Design review of the part built by this model. Coordinates are the model's own, in mm. A direction names the side the tool comes from. Coordinates: 2 decimals unless noted, no trailing zeros. Loops run counter-clockwise (first coordinate to the right, second up) from the corner with the lowest first, then second, coordinate; pieces in that order, holes last. Notation, with made-up numbers: (10, -35.5) - (28, -35.5) arc R21 cw to (28, -20.5) - close; hole circle Ø2 at (41.5, 84). An arc over 180 degrees is marked (long way). Use one line per item in the form item = value. Start each with the question number.
(1) Clearance check with flat-ended pins moving along their axes: pin 1 Ø2 at (y, z) = (1, -17.5) entering from -X; pin 2 Ø2.5 at (x, z) = (20, -113.24) entering from +Y; pin 3 Ø2 at (x, y) = (-18, 2.5) entering from -Z; pin 4 Ø2 at (y, z) = (2.5, -68.5) entering from +X. State where each tip first meets the part, or that it passes through.
(2) Tool access review of faces 1 (the face through (-5.384, 1.972, -121.458)), 2 (the face through (-13.09, 1.97, -1.18)): name each direction out of +Z, -Z, +X, -X, +Y, -Y from which nothing blocks a thin tool from reaching the whole face with its end or side.
(3) Add section B-B (y = 1.1). Count the separate pieces of the cut face and the enclosed holes in it, plus the area to 3 significant figures.
(4) For L1, parallel to X at y = 0.75, z = -66.5; L2, parallel to X at y = 1.95, z = -68.5; L3, parallel to X at y = 0.8, z = -113, list the stretches that pass through material, from the lowest coordinate up.
(5) Add section A-A (z = -79.5). State the section outline as (x, y) points, plus the area to 3 significant figures.
(6) The part is to be moulded in two halves that separate along Z. For faces 3 (the face through (20.922, 1.972, -122.293)), 4 (the face through (8.213, 1.972, -107.86)), 5 (the face through (-23.97, 1.97, -115.82)), 6 (the face through (4.98, 1.97, -43.79)), say which applies: pulls with the +Z half, pulls with the -Z half, needs draft (parallel to the pull), parting line crosses it, or undercut.
```python
from build123d import *

# Parameters (mm, degrees)
BOSS_EXTRUDE1_DEPTH  = 4
M3_CLEARANCE_HOLE1_D = 3.4
SKETCH4_R            = 1.5
CUT_EXTRUDE1_DEPTH   = 135.330995523


with BuildPart() as part:
    # Sketch1 → Boss-Extrude1 (new body)
    with BuildSketch(Plane(origin=(0, 0, 0), x_dir=(1, 0, 0), z_dir=(0, 1, 0))):
        with BuildLine():
            Line((-9.515488572, 0), (9.515488572, 0))
            ThreePointArc((9.515488572, 0), (13.049333225, 1.15108858), (15.227255138, 4.162686012))
            Line((15.227255138, 4.162686012), (21.674585029, 24.205881435))
            ThreePointArc((21.674585029, 24.205881435), (21.904821248, 25.210967753), (21.959569126, 26.240632696))
            Line((21.959569126, 26.240632696), (20.905492982, 58.256025321))
            Line((20.905492982, 58.256025321), (21.026416806, 91.49070067))
            Line((21.026416806, 91.49070067), (23.354507229, 113.886787435))
            ThreePointArc((23.354507229, 113.886787435), (23.340591043, 115.249277617), (23.019622055, 116.573495146))
            Line((23.019622055, 116.573495146), (18.764127525, 128.174177455))
            ThreePointArc((18.764127525, 128.174177455), (16.566422509, 131.027083341), (13.131169609, 132.107831618))
            Line((13.131169609, 132.107831618), (-14.108422678, 132.107831618))
            ThreePointArc((-14.108422678, 132.107831618), (-17.566572488, 131.011014247), (-19.760402704, 128.121564914))
            Line((-19.760402704, 128.121564914), (-23.659003651, 117.179294294))
            ThreePointArc((-23.659003651, 117.179294294), (-23.973087581, 115.802805743), (-23.956822357, 114.391032075))
            Line((-23.956822357, 114.391032075), (-20.971772171, 91.460387024))
            Line((-20.971772171, 91.460387024), (-20.839350394, 58.395973604))
            Line((-20.839350394, 58.395973604), (-22.202521241, 27.066826186))
            ThreePointArc((-22.202521241, 27.066826186), (-22.154511659, 26.005197672), (-21.919959446, 24.968691386))
            Line((-21.919959446, 24.968691386), (-15.227255138, 4.162686012))
            ThreePointArc((-15.227255138, 4.162686012), (-13.049333225, 1.15108858), (-9.515488572, 0))
        make_face()
        Polygon((-13.5, 28.266780853), (-13.5, 45.722835983), (-3.109490994, 36.994808418), align=None, mode=Mode.SUBTRACT)
        Polygon((-10.104794721, 48.094808418), (0, 39.606780853), (10.104794721, 48.094808418), align=None, mode=Mode.SUBTRACT)
        Polygon((13.5, 28.266780853), (13.5, 45.722835983), (3.109490994, 36.994808418), align=None, mode=Mode.SUBTRACT)
        Polygon((0, 34.382835983), (10.104794721, 25.894808418), (-10.104794721, 25.894808418), align=None, mode=Mode.SUBTRACT)
        Polygon((-13.076324897, 19.530410576), (-13.076324897, 13.159093094), (-5.284733567, 16.344751835), align=None, mode=Mode.SUBTRACT)
        Polygon((5.284733567, 16.344751835), (13.076324897, 19.530410576), (13.076324897, 13.159093094), align=None, mode=Mode.SUBTRACT)
        Polygon((-7.79159133, 10.998384586), (0, 14.184043327), (7.79159133, 10.998384586), align=None, mode=Mode.SUBTRACT)
        Polygon((13.75, 102.323235543), (13.75, 124.166381293), (2.828427125, 113.244808418), align=None, mode=Mode.SUBTRACT)
        Polygon((-10.921572875, 99.494808418), (10.921572875, 99.494808418), (0, 110.416381293), align=None, mode=Mode.SUBTRACT)
        Polygon((-13.75, 102.323235543), (-2.828427125, 113.244808418), (-13.75, 124.166381293), align=None, mode=Mode.SUBTRACT)
        Polygon((0, 116.073235543), (-10.921572875, 126.994808418), (10.921572875, 126.994808418), align=None, mode=Mode.SUBTRACT)
        Polygon((-7.79159133, 89.958123907), (-2.137995178, 74.994808418), (-7.79159133, 60.031492928), align=None, mode=Mode.SUBTRACT)
        Polygon((-5.653596152, 54.372882815), (5.653596152, 54.372882815), (0, 69.336198304), align=None, mode=Mode.SUBTRACT)
        Polygon((-5.653596152, 95.616734021), (5.653596152, 95.616734021), (0, 80.653418531), align=None, mode=Mode.SUBTRACT)
        Polygon((7.79159133, 60.031492928), (7.79159133, 89.958123907), (2.137995178, 74.994808418), align=None, mode=Mode.SUBTRACT)
    extrude(amount=BOSS_EXTRUDE1_DEPTH)

    # M3 Clearance Hole1 (through all)
    with Locations(Plane(origin=(0, 4, 0), x_dir=(1, 0, 0), z_dir=(0, 1, 0))):
        with Locations((-7.62, 5.497333735), (7.62, 5.497333735), (20, 113.244808418), (-20, 113.244808418)):
            Hole(M3_CLEARANCE_HOLE1_D / 2)

    # Sketch4 → Cut-Extrude1 (cut, through all)
    with BuildSketch(Plane(origin=(0, 4, 0), x_dir=(1, 0, 0), z_dir=(0, 1, 0))):
        with Locations(Location((-17.653596152, 95.616734021, 0), (0, 0, 270))):
            Circle(SKETCH4_R)
        with Locations(Location((17.653596152, 95.616734021, 0), (0, 0, 270))):
            Circle(SKETCH4_R)
    extrude(amount=-CUT_EXTRUDE1_DEPTH, mode=Mode.SUBTRACT)


solid = part.part
```
Computed values:
q1.pin_1 = -19.84
q1.pin_2 = through
q1.pin_3 = -131.37
q1.pin_4 = 20.95
q2.face_1 = +Y, -Y
q2.face_2 = +Z, -X, +Y, -Y
q3.separate_pieces = 1
q3.enclosed_holes = 21
q3.area = 4,180 mm^2
q4.L1 = -20.87 to -7.79, -5.35 to -1.07, 1.07 to 5.35, 7.79 to 20.94
q4.L2 = -20.88 to -7.79, -4.59 to -0.32, 0.32 to 4.59, 7.79 to 20.94
q4.L3 = -23.78 to -21.68, -18.32 to -13.75, -3.07 to 3.07, 13.75 to 18.32, 21.68 to 23.26
q5.outline = (-20.92, 0) - (-7.79, 0) - (-7.79, 4) - (-20.92, 4) - close; (-3.84, 0) - (3.84, 0) - (3.84, 4) - (-3.84, 4) - close; (7.79, 0) - (20.98, 0) - (20.98, 4) - (7.79, 4) - close
q5.area = 136 mm^2
q6.face_3 = pulls with the -Z half
q6.face_4 = undercut
q6.face_5 = parting line crosses it
q6.face_6 = undercut
